```python
from build123d import *

# Parameters (mm, degrees)
F1_DEPTH = 22.5
F3_DEPTH = 15
F4_W     = 25.6565664813
F4_H     = 15.121226953
F5_DEPTH = 5
F6_R     = 5
F8_DEPTH = 46.9898349885
F9_R     = 1


with BuildPart() as f1:
    # F0 (on Top) → F1 (new body)
    with BuildSketch(Plane.XY):
        Polygon((0, 47), (0, 0), (45.5, 0), (45.9890725419, 45.997400014), align=None)
    extrude(amount=F1_DEPTH)

    # F2 (on Top) → F3 (cut)
    with BuildSketch(Plane.XY):
        Polygon((1.5, 33.5), (1.5, 1.5), (44.0079360013, 1.5), (44.4654638771, 44.5306159486), (0, 45.5), (0, 33.5), align=None)
    extrude(amount=F3_DEPTH, mode=Mode.SUBTRACT)

    # F4 (on face) → F5 (cut)
    with BuildSketch(Plane(origin=(0, 0, 15), x_dir=(1, 0, 0), z_dir=(0, 0, -1))):
        with Locations((27.3282832406, -23.0606134765)):
            Rectangle(F4_W, F4_H)
    extrude(amount=-F5_DEPTH, mode=Mode.SUBTRACT)

    # F6
    f6_edges = [f1.edges().sort_by_distance(p)[0] for p in [
        (14.5, 30.621227, 17.5),
        (40.156566, 30.621227, 17.5),
        (14.5, 15.5, 17.5),
        (40.156566, 15.5, 17.5),
    ]]
    fillet(f6_edges, radius=F6_R)

    # F7 (on face) → F8 (cut, through all)
    with BuildSketch(Plane(origin=(1.0241522892, 46.9776726293, 0), x_dir=(-0.9997624466, 0.0217956519, 0), z_dir=(0.0217956519, 0.9997624466, 0))):
        with BuildLine():
            Line((-16.9756043621, 0), (-8.9756043621, 0))
            Line((-8.9756043621, 0), (-8.9756043621, 9))
            ThreePointArc((-8.9756043621, 9), (-9.8542840186, 11.1213203436), (-11.9756043621, 12))
            Line((-11.9756043621, 12), (-13.9756043621, 12))
            ThreePointArc((-13.9756043621, 12), (-16.0969247057, 11.1213203436), (-16.9756043621, 9))
            Line((-16.9756043621, 9), (-16.9756043621, 0))
        make_face()
        with BuildLine():
            Line((-34.9756043621, 0), (-24.9756043621, 0))
            Line((-24.9756043621, 0), (-24.9756043621, 9))
            ThreePointArc((-24.9756043621, 9), (-25.8542840186, 11.1213203436), (-27.9756043621, 12))
            Line((-27.9756043621, 12), (-31.9756043621, 12))
            ThreePointArc((-31.9756043621, 12), (-34.0969247057, 11.1213203436), (-34.9756043621, 9))
            Line((-34.9756043621, 9), (-34.9756043621, 0))
        make_face()
    extrude(amount=-F8_DEPTH, mode=Mode.SUBTRACT)

    # F9
    f9_edges = [f1.edges().sort_by_distance(p)[0] for p in [
        (1.5, 1.5, 7.5),
        (44.007936, 1.5, 7.5),
        (44.465464, 44.530616, 7.5),
    ]]
    fillet(f9_edges, radius=F9_R)


solid = f1.part
```
Here's how the part is built. I have some questions about the finished solid (model axes, mm). A direction names the side the tool comes from. Coordinates: 2 decimals unless noted, no trailing zeros. Write each loop counter-clockwise with the first axis right and the second up, starting at its lowest first coordinate (ties: lowest second). Pieces come first, ordered by that corner, then holes. Notation, with made-up numbers: (54, -36) -> (67, -36) arc R33 ccw to (67, 1) -> close; hole circle Ø2 at (43, -24.5). An arc over 180 degrees is marked (long way). Use a Markdown table: item, result. Add a question column.
(1) We'd pull the mould along Y, two halves only. Please class faces 1 (the flat face through (14, 46, 12)), 2 (the cylindrical face through (38.73, 29.12, 17.54)): +Y half, -Y half, draft (parallel to the pull), parting line (faces both ways), or undercut.
(2) If we section it at D-D, the plane x = 22: Write out the boundary of the cut face in (y, z), and give its area (3 significant figures).
(3) Please list where these lines run through material, in increasing order: line 1 (Z direction, x = 31, y = 21); line 2 (Z direction, x = 33, y = 39.5); line 3 (X direction, y = 28.5, z = 14).
(4) If we section it at B-B, the plane z = 14: Write out the boundary of the cut face in (x, y) (3 decimals).
(5) If we section it at A-A, the plane z = 6.5: State how many separate pieces and enclosed holes the cut face has, and give its area (3 significant figures).
(6) If we section it at C-C, the plane y = 28: Write out the boundary of the cut face in (x, z), and give its area (3 significant figures).
(7) I'm going to push flat-ended pins straight in: P1, Ø1.5, axis at x = 27, z = 17.5, coming from the +Y side; P2, Ø0.5, axis at x = 29, y = 1, coming from the -Z side; P3, Ø2.5, axis at y = 22.5, z = 18.5, coming from the +X side. Where does each tip first touch, or does it pass through?
(8) For faces 3 (the flat face through (1, 33.5, 7)), 4 (the cylindrical face through (9.85, 0.78, 11.1)), which set-ups out of +Z, -Z, +X, -X, +Y, -Y let a thin tool reach every point of the face, with its end or its side?
Outcome:
| question | item | result |
|---|---|---|
| 1 | face 1 | draft |
| 1 | face 2 | undercut |
| 2 | outline | (0, 0) -> (1.5, 0) -> (1.5, 15) -> (15.5, 15) -> (15.5, 20) -> (30.62, 20) -> (30.62, 15) -> (45.02, 15) -> (45.02, 0) -> (46.52, 0) -> (46.52, 22.5) -> (0, 22.5) -> close |
| 2 | area | 318 mm^2 |
| 3 | line 1 | z = 20 to 22.5 |
| 3 | line 2 | z = 15 to 22.5 |
| 3 | line 3 | x = 0 to 1.5, 44.3 to 45.8 |
| 4 | outline | (0, 0) -> (45.5, 0) -> (45.989, 45.997) -> (0, 47) -> (0, 45.5) -> (43.477, 44.552) arc R1 cw to (44.455, 43.542) -> (44.018, 2.489) arc R1 cw to (43.019, 1.5) -> (2.5, 1.5) arc R1 cw to (1.5, 2.5) -> (1.5, 33.5) -> (0, 33.5) -> close |
| 5 | separate pieces | 5 |
| 5 | enclosed holes | 0 |
| 5 | area | 197 mm^2 |
| 6 | outline | (0, 0) -> (1.5, 0) -> (1.5, 15) -> (15.1, 15) -> (15.1, 20) -> (39.55, 20) -> (39.55, 15) -> (44.29, 15) -> (44.29, 0) -> (45.8, 0) -> (45.8, 22.5) -> (0, 22.5) -> close |
| 6 | area | 266 mm^2 |
| 7 | P1 | stops at y = 46.43 |
| 7 | P2 | stops at z = 12 |
| 7 | P3 | stops at x = 45.75 |
| 8 | face 3 | -Z, -X |
| 8 | face 4 | -Z, -Y |
